from build123d import *

# Parameters (mm, degrees)
F0_W     = 45
F0_H     = 20.5
F1_DEPTH = 1.6
F2_R     = 8
F3_DEPTH = 16


with BuildPart() as f1:
    # F0 (on Front) → F1 (new body)
    with BuildSketch(Plane.XZ):
        Rectangle(F0_W, F0_H)
    extrude(amount=F1_DEPTH)

    # F2 (on Front) → F3 (join)
    with BuildSketch(Plane.XZ):
        with Locations((-13.5, 0)):
            Circle(F2_R)
        with BuildLine():
            ThreePointArc((21.5, 0), (13.5, 8), (5.5, 0))
            ThreePointArc((5.5, 0), (13.5, -8), (21.5, 0))
        make_face()
    extrude(amount=F3_DEPTH)


solid = f1.part
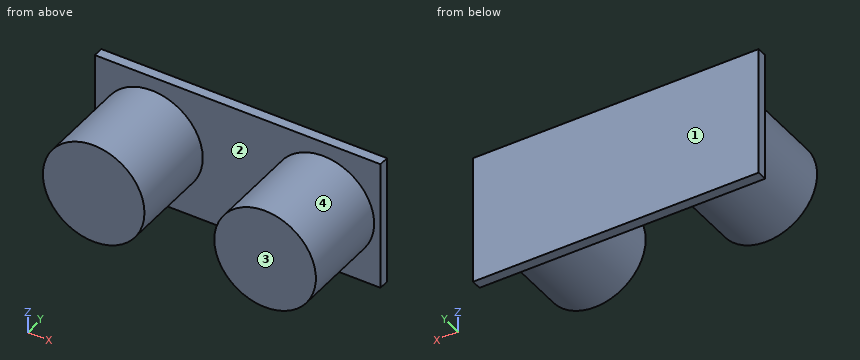
Verification items for the finished model (mm, model axes). Face numbers are marked on the shaded views. A direction names the side the tool comes from. Give positions to 0.01 mm unless a question says otherwise; leave off trailing zeros. Loops run counter-clockwise (first coordinate to the right, second up) from the corner with the lowest first, then second, coordinate; pieces in that order, holes last. Notation, with made-up numbers: (-17, -16.75) - (25, -16.75) arc R23 ccw to (25, 15.25) - close; hole circle Ø1 at (89, 64.25). An arc over 180 degrees is marked (long way). Write item = value, one per line. Start each with the question number.
Q1. Thickness scan on line 1 (Y direction, x = -18, z = -8.25); line 2 (X direction, y = -2, z = 6.5); line 3 (X direction, y = -9.5, z = 3.5). Record the ranges inside material, lowest first.
Q2. Cross-section at B-B, the plane y = -8. Enter the section's corners in (x, z), and give its area (3 significant figures).
Q3. Tool access check on the marked faces 1 and 2. Record the directions out of +Z, -Z, +X, -X, +Y, -Y that give a thin tool (end or side, any length) a straight path to the whole face; none if there is none.
Q4. Cross-section at C-C, the plane x = -13.5. Enter the section's corners in (y, z), and give its area (3 significant figures).
Q5. Depth check by flat-ended pin: P1, Ø3, axis at x = 5, z = -5, coming from the -Y side; P2, Ø5, axis at x = 15.5, y = -12.5, coming from the -Z side; P3, Ø4, axis at y = -9.5, z = 1.5, coming from the -X side. Enter the tip coordinate at first touch or a pass-through.
Q6. Cross-section at A-A, the plane z = 0. Enter the section's corners in (x, y), and give its area (3 significant figures).
Q7. Cross-section at D-D, the plane z = -8.75. Enter the section's corners in (x, y), and give its area (3 significant figures).
Q8. Mould release check, pull along X, two halves, no side actions. Record for the marked faces 3 and 4: released by +X, released by -X, zero draft, split by the parting line, or undercut.
Answer key:
q1.line_1 = -1.6 to 0
q1.line_2 = -18.16 to -8.84, 8.84 to 18.16
q1.line_3 = -20.69 to -6.31, 6.31 to 20.69
q2.outline = circle Ø16 at (-13.5, 0); circle Ø16 at (13.5, 0)
q2.area = 402 mm^2
q3.face_1 = +Z, -Z, +X, -X, +Y
q3.face_2 = -Y
q4.outline = (-16, -8) - (-1.6, -8) - (-1.6, -10.25) - (0, -10.25) - (0, 10.25) - (-1.6, 10.25) - (-1.6, 8) - (-16, 8) - close
q4.area = 263 mm^2
q5.P1 = -1.6
q5.P2 = -8
q5.P3 = -21.5
q6.outline = (-22.5, -1.6) - (-21.5, -1.6) - (-21.5, -16) - (-5.5, -16) - (-5.5, -1.6) - (5.5, -1.6) - (5.5, -16) - (21.5, -16) - (21.5, -1.6) - (22.5, -1.6) - (22.5, 0) - (-22.5, 0) - close
q6.area = 533 mm^2
q7.outline = (-22.5, -1.6) - (22.5, -1.6) - (22.5, 0) - (-22.5, 0) - close
q7.area = 72.0 mm^2
q8.face_3 = zero draft
q8.face_4 = undercut
